Here's how the part is built. I have some questions about the finished solid (model axes, mm). Face numbers are marked on the shaded views. Give positions to 0.01 mm unless a question says otherwise; leave off trailing zeros. Write each loop counter-clockwise with the first axis right and the second up, starting at its lowest first coordinate (ties: lowest second). Pieces come first, ordered by that corner, then holes. Notation, with made-up numbers: (-12, 69.25) -> (9, 69.25) arc R15 cw to (9, 73.25) -> close; hole circle Ø3 at (81, -32.75). An arc over 180 degrees is marked (long way). Use CSV: the item, a comma, the result in double quotes. Start each with the question number.
(1) Suppose I cut it at A-A on y = 63.55. List the corners of the cut face in (x, z) for me.
(2) I need wall thicknesses on L1, parallel to Y at x = 60, z = 1.4; L2, parallel to Y at x = 14, z = 1.75; L3, parallel to X at y = 72.5, z = 4. Which ranges of each line are inside material? Lowest first, please. Write a range as [from, to].
(3) If we mould it in two halves opening along Y, with no side actions, what happens to the marked faces 1, 2, 3 and 4? For each: pulls with the +Y half, pulls with the -Y half, needs draft (parallel to the pull), parting line crosses it, or undercut.
(4) Suppose I cut it at D-D on z = 1.75. Give the number of separate pieces and of enclosed holes in the cut face, plus the area to 3 significant figures.
(5) Suppose I cut it at B-B on y = 40. List the corners of the cut face in (x, z) for me, plus the area to 3 significant figures.
(6) Suppose I cut it at C-C on y = 55.5. List the corners of the cut face in (x, z) for me, plus the area to 3 significant figures.
(7) For pin 1 Ø3 at (x, y) = (30, 6.5) entering from +Z, with a flat end and sliding along its axis, tell me the tip position at first contact or that it passes through.
from build123d import *

# Parameters (mm, degrees)
CROQUIS1_W              = 75
CROQUIS1_H              = 80
SALIENTE_EXTRUIR1_DEPTH = 6
CORTAR_EXTRUIR1_DEPTH   = 7
REDONDEO1_R             = 12
CROQUIS3_R              = 2
CORTAR_EXTRUIR2_DEPTH   = 7


with BuildPart() as part:
    # Croquis1 → Saliente-Extruir1 (new body)
    with BuildSketch(Plane.XY):
        with Locations((37.5, 40)):
            Rectangle(CROQUIS1_W, CROQUIS1_H)
    extrude(amount=SALIENTE_EXTRUIR1_DEPTH)

    # Croquis2 → Cortar-Extruir1 (cut, through all)
    with BuildSketch(Plane(origin=(0, 0, 0), x_dir=(-1, 0, 0), z_dir=(0, 0, -1))):
        with BuildLine():
            Line((-36, 28.9), (-42, 28.9))
            ThreePointArc((-42, 28.9), (-53.1, 40), (-42, 51.1))
            Line((-42, 51.1), (-36, 51.1))
            ThreePointArc((-36, 51.1), (-24.9, 40), (-36, 28.9))
        make_face()
        with BuildLine():
            Line((-20.5, 22.85), (-26.5, 22.85))
            ThreePointArc((-26.5, 22.85), (-28.15, 24.5), (-26.5, 26.15))
            Line((-26.5, 26.15), (-20.5, 26.15))
            ThreePointArc((-20.5, 26.15), (-18.85, 24.5), (-20.5, 22.85))
        make_face()
        with BuildLine():
            Line((-51.5, 53.85), (-57.5, 53.85))
            ThreePointArc((-57.5, 53.85), (-59.15, 55.5), (-57.5, 57.15))
            Line((-57.5, 57.15), (-51.5, 57.15))
            ThreePointArc((-51.5, 57.15), (-49.85, 55.5), (-51.5, 53.85))
        make_face()
        with BuildLine():
            Line((-51.5, 22.85), (-57.5, 22.85))
            ThreePointArc((-57.5, 22.85), (-59.15, 24.5), (-57.5, 26.15))
            Line((-57.5, 26.15), (-51.5, 26.15))
            ThreePointArc((-51.5, 26.15), (-49.85, 24.5), (-51.5, 22.85))
        make_face()
        with BuildLine():
            Line((-20.5, 53.85), (-26.5, 53.85))
            ThreePointArc((-26.5, 53.85), (-28.15, 55.5), (-26.5, 57.15))
            Line((-26.5, 57.15), (-20.5, 57.15))
            ThreePointArc((-20.5, 57.15), (-18.85, 55.5), (-20.5, 53.85))
        make_face()
        with BuildLine():
            Line((-12.45, 13.85), (-18.45, 13.85))
            ThreePointArc((-18.45, 13.85), (-21.05, 16.45), (-18.45, 19.05))
            Line((-18.45, 19.05), (-12.45, 19.05))
            ThreePointArc((-12.45, 19.05), (-9.85, 16.45), (-12.45, 13.85))
        make_face()
        with BuildLine():
            Line((-59.55, 13.85), (-65.55, 13.85))
            ThreePointArc((-65.55, 13.85), (-68.15, 16.45), (-65.55, 19.05))
            Line((-65.55, 19.05), (-59.55, 19.05))
            ThreePointArc((-59.55, 19.05), (-56.95, 16.45), (-59.55, 13.85))
        make_face()
        with BuildLine():
            Line((-12.45, 60.95), (-18.45, 60.95))
            ThreePointArc((-18.45, 60.95), (-21.05, 63.55), (-18.45, 66.15))
            Line((-18.45, 66.15), (-12.45, 66.15))
            ThreePointArc((-12.45, 66.15), (-9.85, 63.55), (-12.45, 60.95))
        make_face()
        with BuildLine():
            Line((-59.55, 60.95), (-65.55, 60.95))
            ThreePointArc((-65.55, 60.95), (-68.15, 63.55), (-65.55, 66.15))
            Line((-65.55, 66.15), (-59.55, 66.15))
            ThreePointArc((-59.55, 66.15), (-56.95, 63.55), (-59.55, 60.95))
        make_face()
    extrude(amount=-CORTAR_EXTRUIR1_DEPTH, mode=Mode.SUBTRACT)

    # Redondeo1
    redondeo1_edges = [part.edges().sort_by_distance(p)[0] for p in [
        (0, 80, 3),
        (0, 0, 3),
    ]]
    fillet(redondeo1_edges, radius=REDONDEO1_R)

    # Croquis3 → Cortar-Extruir2 (cut, through all)
    with BuildSketch(Plane(origin=(0, 0, 0), x_dir=(-1, 0, 0), z_dir=(0, 0, -1))):
        with Locations((-60, 6.5)):
            Circle(CROQUIS3_R)
        with Locations((-30, 6.5)):
            Circle(CROQUIS3_R)
        with Locations((-60, 73.5)):
            Circle(CROQUIS3_R)
        with Locations((-30, 73.5)):
            Circle(CROQUIS3_R)
    extrude(amount=-CORTAR_EXTRUIR2_DEPTH, mode=Mode.SUBTRACT)


solid = part.part
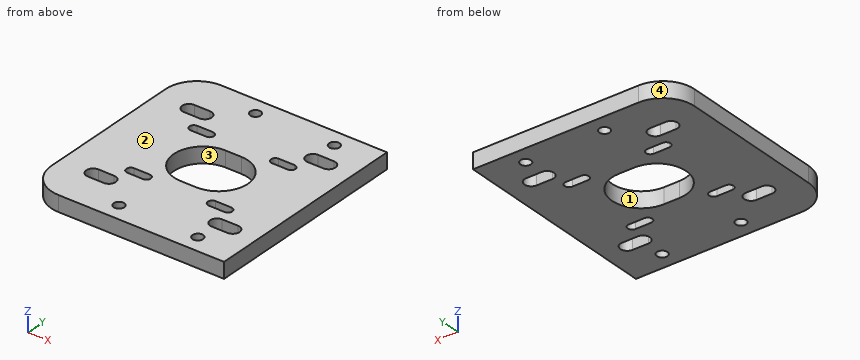
Geometry says:
1,outline,"(0, 0) -> (9.85, 0) -> (9.85, 6) -> (0, 6) -> close; (21.05, 0) -> (56.95, 0) -> (56.95, 6) -> (21.05, 6) -> close; (68.15, 0) -> (75, 0) -> (75, 6) -> (68.15, 6) -> close"
2,L1,"[0, 4.5], [8.5, 13.85], [19.05, 60.95], [66.15, 71.5], [75.5, 80]"
2,L2,"[0, 13.85], [19.05, 60.95], [66.15, 80]"
2,L3,"[0.88, 28.27], [31.73, 58.27], [61.73, 75]"
3,face 1,"undercut"
3,face 2,"needs draft"
3,face 3,"undercut"
3,face 4,"pulls with the +Y half"
4,separate pieces,"1"
4,enclosed holes,"13"
4,area,"5,040 mm²"
5,outline,"(0, 0) -> (24.9, 0) -> (24.9, 6) -> (0, 6) -> close; (53.1, 0) -> (75, 0) -> (75, 6) -> (53.1, 6) -> close"
5,area,"281 mm²"
6,outline,"(0, 0) -> (18.85, 0) -> (18.85, 6) -> (0, 6) -> close; (28.15, 0) -> (49.85, 0) -> (49.85, 6) -> (28.15, 6) -> close; (59.15, 0) -> (75, 0) -> (75, 6) -> (59.15, 6) -> close"
6,area,"338 mm²"
7,pin 1,"through"
